Verification items for the finished model (mm, model axes). Round coordinates to 2 decimals unless told otherwise and drop trailing zeros. Write each loop counter-clockwise with the first axis right and the second up, starting at its lowest first coordinate (ties: lowest second). Pieces come first, ordered by that corner, then holes. Notation, with made-up numbers: M -39.5,89 L -3.5,89 A9 ccw -3.5,105 Z; hole C 55.5,53.5 d5. An arc over 180 degrees is marked long. Answer in a Markdown table with one row per item. Add a question column.
1. Material ranges on probe 1 along X at (y, z) = (3, 25); probe 2 along X at (y, z) = (6.75, 70), recorded low to high.
2. Sectioned sample at C-C on z = -70. Record the cut outline in (x, y) (3 decimals), plus the area to 3 significant figures.
3. Sectioned sample at D-D on y = 7.5. Count the separate pieces of the cut face and the enclosed holes in it, plus the area to 3 significant figures.
4. Sectioned sample at B-B on z = 85. Record the cut outline in (x, y).
5. Go/stop test with flat-tipped pins: pin 1 Ø5 at (y, z) = (7, 10.5) entering from -X; pin 2 Ø4 at (y, z) = (5.5, -16.5) entering from +X. Record where each tip stops, or that it passes through.
6. Sectioned sample at A-A on x = 70. Record the cut outline in (y, z) (3 decimals).
```python
from build123d import *

# Parameters (mm, degrees)
BOSS_EXTRUDE1_DEPTH            = 10
M6_CLEARANCE_HOLE1_D           = 6.6
M6_CLEARANCE_HOLE1_CSINK_D     = 6.65
M6_CLEARANCE_HOLE1_CSINK_ANGLE = 100


with BuildPart() as part:
    # Sketch1 → Boss-Extrude1 (new body)
    with BuildSketch(Plane(origin=(0, 0, 0), x_dir=(1, 0, 0), z_dir=(0, 1, 0))):
        Polygon((-50, 80), (50, 80), (50, 100), (100, 100), (100, 50), (80, 50), (80, -50), (100, -50), (100, -100), (50, -100), (50, -80), (-50, -80), (-50, -100), (-100, -100), (-100, -50), (-80, -50), (-80, 50), (-100, 50), (-100, 100), (-50, 100), align=None)
    extrude(amount=BOSS_EXTRUDE1_DEPTH)

    # M6 Clearance Hole1 (through all)
    with Locations(Plane(origin=(0, 10, 0), x_dir=(1, 0, 0), z_dir=(0, 1, 0))):
        with Locations((-70, -25), (-70, 25), (-25, 70), (25, 70), (70, 25), (70, -25), (-25, -70), (25, -70)):
            CounterSinkHole(M6_CLEARANCE_HOLE1_D / 2, M6_CLEARANCE_HOLE1_CSINK_D / 2, counter_sink_angle=M6_CLEARANCE_HOLE1_CSINK_ANGLE)


solid = part.part
```
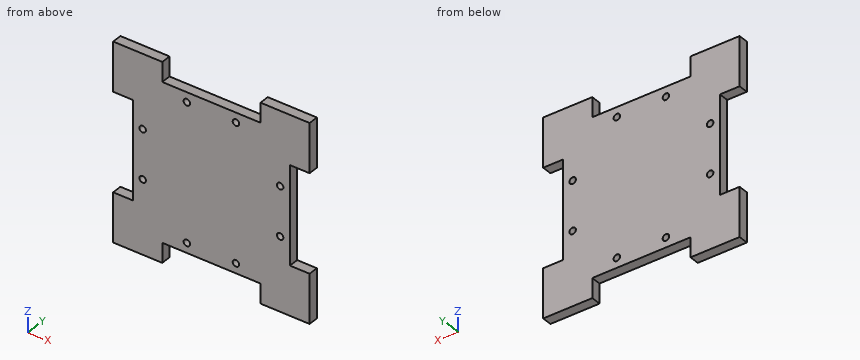
Geometry check:
| question | item | result |
|---|---|---|
| 1 | probe 1 | x = -80 to -73.3, -66.7 to 66.7, 73.3 to 80 |
| 1 | probe 2 | x = -100 to -28.3, -21.7 to 21.7, 28.3 to 100 |
| 2 | outline | M -100,0 L -28.3,0 L -28.3,9.979 L -28.325,10 L -100,10 Z; M -21.7,0 L 21.7,0 L 21.7,9.979 L 21.675,10 L -21.675,10 L -21.7,9.979 Z; M 28.3,0 L 100,0 L 100,10 L 28.325,10 L 28.3,9.979 Z |
| 2 | area | 1,870 mm2 |
| 3 | separate pieces | 1 |
| 3 | enclosed holes | 8 |
| 3 | area | 31,700 mm2 |
| 4 | outline | M -100,0 L -50,0 L -50,10 L -100,10 Z; M 50,0 L 100,0 L 100,10 L 50,10 Z |
| 5 | pin 1 | stops at x = -80 |
| 5 | pin 2 | stops at x = 80 |
| 6 | outline | M 0,-100 L 10,-100 L 10,-28.325 L 9.979,-28.3 L 0,-28.3 Z; M 0,-21.7 L 9.979,-21.7 L 10,-21.675 L 10,21.675 L 9.979,21.7 L 0,21.7 Z; M 0,28.3 L 9.979,28.3 L 10,28.325 L 10,100 L 0,100 Z |
